Source: CAD feature listing. Evaluate the final solid. Frame: model axes, mm. Give positions to 0.01 mm unless a question says otherwise; leave off trailing zeros. Order: outer loops, then holes, each group sorted by start corner. A loop starts at its lowest first (then second) coordinate and runs counter-clockwise, first axis right, second up. Notation, with made-up numbers: M -9,-9.5 L 50,-9.5 A27 ccw 50,11.5 Z; hole C 56.25,69 d8. An arc over 180 degrees is marked long. Answer in a Markdown table with one row per item. Add a question column.
(1) Section query A-A, the plane z = 15.25. Return loops of the section in (x, y) (3 decimals).
(2) Material intervals for line 1 along X through (y, z) = (25, -15.25) (3 decimals); line 2 along Z through (x, y) = (12.25, 18.75) (3 decimals); line 3 along Z through (x, y) = (13, 25.5), sorted ascending.
(3) Section query D-D, the plane y = 21.5. Return loops of the section in (x, z) (3 decimals), plus the area to 3 significant figures.
(4) Section query B-B, the plane x = 12.25. Return loops of the section in (y, z) (3 decimals).
(5) Section query C-C, the plane y = 29. Return loops of the section in (x, z) (3 decimals).
(6) Mould query, pull axis X, two halves, no side actions, for faces 1 (the face through (-11.24, 22.6, 13.67)), 2 (the face through (0, 22, 18)), 3 (the face through (-15, 29, 0)). Classes: pulls with the +X half, pulls with the -X half, needs draft (parallel to the pull), parting line crosses it, or undercut.
(7) Pin query (flat end, axial travel): P1, Ø2, axis at x = 5, z = -6.5, coming from the -Y side. Return the tip coordinate at first contact, or that it passes through.
from build123d import *

# Parameters (mm, degrees)
SKETCH1_W           = 30
SKETCH1_H           = 36
BOSS_EXTRUDE1_DEPTH = 30
SKETCH3_R           = 12.375
CUT_EXTRUDE1_DEPTH  = 40
SKETCH5_R           = 1.875
CUT_EXTRUDE2_DEPTH  = 40
CUT_EXTRUDE3_START  = 15
SKETCH7_W           = 36
SKETCH7_H           = 15
CUT_EXTRUDE3_DEPTH  = 31


with BuildPart() as part:
    # Sketch1 → Boss-Extrude1 (new body)
    with BuildSketch(Plane(origin=(0, 0, 0), x_dir=(1, 0, 0), z_dir=(0, 1, 0))):
        Rectangle(SKETCH1_W, SKETCH1_H)
    extrude(amount=BOSS_EXTRUDE1_DEPTH)

    # Sketch3 → Cut-Extrude1 (cut)
    with BuildSketch(Plane(origin=(15, 0, 0), x_dir=(0, 0, -1), z_dir=(1, 0, 0))):
        with Locations((0, 15)):
            Circle(SKETCH3_R)
    extrude(amount=-CUT_EXTRUDE1_DEPTH, mode=Mode.SUBTRACT)

    # Sketch5 → Cut-Extrude2 (cut)
    with BuildSketch(Plane(origin=(0, 30, 0), x_dir=(1, 0, 0), z_dir=(0, 1, 0))):
        with Locations((-12.25, 15.25)):
            Circle(SKETCH5_R)
        with Locations((-12.25, -15.25)):
            Circle(SKETCH5_R)
        with Locations((12.25, -15.25)):
            Circle(SKETCH5_R)
        with Locations((12.25, 15.25)):
            Circle(SKETCH5_R)
    extrude(amount=-CUT_EXTRUDE2_DEPTH, mode=Mode.SUBTRACT)

    # Sketch7 → Cut-Extrude3 (cut, through all)
    with BuildSketch(Plane(origin=(0, 0, 0), x_dir=(0, 0, -1), z_dir=(1, 0, 0)).offset(CUT_EXTRUDE3_START)):
        with Locations((0, 7.5)):
            Rectangle(SKETCH7_W, SKETCH7_H)
    extrude(amount=-CUT_EXTRUDE3_DEPTH, mode=Mode.SUBTRACT)


solid = part.part
Values follow:
| question | item | result |
|---|---|---|
| 1 | outline | M -15,15 L -14.125,15 L -14.125,30 L -15,30 Z; M -10.375,15 L 10.375,15 L 10.375,30 L -10.375,30 Z; M 14.125,15 L 15,15 L 15,30 L 14.125,30 Z |
| 2 | line 1 | x = -15 to -14.125, -10.375 to 10.375, 14.125 to 15 |
| 2 | line 2 | z = -18 to -17.125, -13.375 to -11.793, 11.793 to 13.375, 17.125 to 18 |
| 2 | line 3 | z = -18 to -16.97, -13.53 to -6.55, 6.55 to 13.53, 16.97 to 18 |
| 3 | outline | M -15,-18 L 15,-18 L 15,-10.53 L -15,-10.53 Z; M -15,10.53 L 15,10.53 L 15,18 L -15,18 Z; hole C -12.25,-15.25 d3.75; hole C -12.25,15.25 d3.75; hole C 12.25,-15.25 d3.75; hole C 12.25,15.25 d3.75 |
| 3 | area | 404 mm² |
| 4 | outline | M 15,-18 L 30,-18 L 30,-17.125 L 15,-17.125 Z; M 15,-13.375 L 30,-13.375 L 30,13.375 L 15,13.375 L 15,12.375 A12.375 cw 15,-12.375 Z; M 15,17.125 L 30,17.125 L 30,18 L 15,18 Z |
| 5 | outline | M -15,-18 L 15,-18 L 15,18 L -15,18 Z; hole C -12.25,-15.25 d3.75; hole C -12.25,15.25 d3.75; hole C 12.25,-15.25 d3.75; hole C 12.25,15.25 d3.75 |
| 6 | face 1 | undercut |
| 6 | face 2 | needs draft |
| 6 | face 3 | pulls with the -X half |
| 7 | P1 | stops at y = 24.84 |
